from build123d import *

# Parameters (mm, degrees)
BOSS_EXTRUDE1_DEPTH = 4
SKETCH2_R           = 1
CUT_EXTRUDE1_DEPTH  = 5


with BuildPart() as part:
    # Sketch1 → Boss-Extrude1 (new body)
    with BuildSketch(Plane(origin=(0, 0, 0), x_dir=(1, 0, 0), z_dir=(0, 1, 0))):
        with BuildLine():
            Line((-32, -13), (32, -13))
            ThreePointArc((32, -13), (34.121320344, -12.121320344), (35, -10))
            Line((35, -10), (35, 10))
            ThreePointArc((35, 10), (34.121320344, 12.121320344), (32, 13))
            Line((32, 13), (-32, 13))
            ThreePointArc((-32, 13), (-34.121320344, 12.121320344), (-35, 10))
            Line((-35, 10), (-35, -10))
            ThreePointArc((-35, -10), (-34.121320344, -12.121320344), (-32, -13))
        make_face()
        with BuildLine():
            Line((-26.749817226, -6), (26.749817226, -6))
            ThreePointArc((26.749817226, -6), (28.871137569, -5.121320344), (29.749817226, -3))
            Line((29.749817226, -3), (29.749817226, 3))
            ThreePointArc((29.749817226, 3), (28.871137569, 5.121320344), (26.749817226, 6))
            Line((26.749817226, 6), (-26.749817226, 6))
            ThreePointArc((-26.749817226, 6), (-28.871137569, 5.121320344), (-29.749817226, 3))
            Line((-29.749817226, 3), (-29.749817226, -3))
            ThreePointArc((-29.749817226, -3), (-28.871137569, -5.121320344), (-26.749817226, -6))
        make_face(mode=Mode.SUBTRACT)
        with BuildLine():
            Line((-28.749817226, 11.5), (28.749817226, 11.5))
            ThreePointArc((28.749817226, 11.5), (29.456924007, 11.207106781), (29.749817226, 10.5))
            Line((29.749817226, 10.5), (29.749817226, 9.5))
            ThreePointArc((29.749817226, 9.5), (29.456924007, 8.792893219), (28.749817226, 8.5))
            Line((28.749817226, 8.5), (-28.749817226, 8.5))
            ThreePointArc((-28.749817226, 8.5), (-29.456924007, 8.792893219), (-29.749817226, 9.5))
            Line((-29.749817226, 9.5), (-29.749817226, 10.5))
            ThreePointArc((-29.749817226, 10.5), (-29.456924007, 11.207106781), (-28.749817226, 11.5))
        make_face(mode=Mode.SUBTRACT)
        with BuildLine():
            Line((-29.749817226, -10.5), (-29.749817226, -9.5))
            ThreePointArc((-29.749817226, -9.5), (-29.456924007, -8.792893219), (-28.749817226, -8.5))
            Line((-28.749817226, -8.5), (28.749817226, -8.5))
            ThreePointArc((28.749817226, -8.5), (29.456924007, -8.792893219), (29.749817226, -9.5))
            Line((29.749817226, -9.5), (29.749817226, -10.5))
            ThreePointArc((29.749817226, -10.5), (29.456924007, -11.207106781), (28.749817226, -11.5))
            Line((28.749817226, -11.5), (-28.749817226, -11.5))
            ThreePointArc((-28.749817226, -11.5), (-29.456924007, -11.207106781), (-29.749817226, -10.5))
        make_face(mode=Mode.SUBTRACT)
    extrude(amount=BOSS_EXTRUDE1_DEPTH)

    # Sketch2 → Cut-Extrude1 (cut)
    with BuildSketch(Plane(origin=(35, 0, 0), x_dir=(0, 0, -1), z_dir=(1, 0, 0))):
        with Locations((-8, 2)):
            Circle(SKETCH2_R)
        with Locations((8, 2)):
            Circle(SKETCH2_R)
    extrude(amount=-CUT_EXTRUDE1_DEPTH, mode=Mode.SUBTRACT)


solid = part.part
The model under review builds one solid part; all positions refer to its coordinate system, in mm. A direction names the side the tool comes from. Give positions to 0.01 mm unless a question says otherwise; leave off trailing zeros. Write each loop counter-clockwise with the first axis right and the second up, starting at its lowest first coordinate (ties: lowest second). Pieces come first, ordered by that corner, then holes. Notation, with made-up numbers: M 88.5,84.5 L 143.5,84.5 A30 ccw 143.5,107.5 Z; hole C 30,-28.75 d11. An arc over 180 degrees is marked long. One line per question, with ' | ' between items. Start each with the question number.
Item 1: Wall thickness on line 1 (Z direction, x = 13, y = 2.1); line 2 (Y direction, x = 32.4, z = 8); line 3 (X direction, y = 3.1, z = -3.25): over which ranges is each line inside the solid? List them lowest first. Write a range as from..to.
Item 2: We need section D-D on y = 2. Give the number of separate pieces and of enclosed holes in the cut face, plus the area to 3 significant figures.
Item 3: For pin 1 (1.6 mm diameter, centred on y = 2, z = -8, fed in from +X), flat-tipped, find the tip position at first contact; note if it passes through.
Item 4: For faces 1 (the cylindrical face through (-34.14, 1.97, 12.1)), 2 (the flat face through (0, 2, -8.5)), list the 3-axis set-ups (+Z, -Z, +X, -X, +Y, -Y) from which the entire face can be reached by the end or side of a thin tool; tool diameter is ignored.
Item 5: We need section A-A on x = 19. Write out the cut boundary in (y, z).
Item 6: Draft analysis for pull direction Y (two halves, no side actions). For faces 3 (the flat face through (30, 2, -8)), 4 (the flat face through (0, 4, 8)), 5 (the flat face through (30, 2, 8)), 6 (the flat face through (35, 2, 0)), state which applies: released by +Y, released by -Y, zero draft, split by the parting line, or undercut.
Item 7: We need section B-B on z = -2. Write out the cut boundary in (x, y).
Item 8: We need section C-C on x = -28. Write out the cut boundary in (y, z).
Results found:
1) line 1: z = -13..-11.5, -8.5..-6, 6..8.5, 11.5..13 | line 2: y = 0..1, 3..4 | line 3: x = -35..-29.74, 29.74..35
2) separate pieces: 1 | enclosed holes: 3 | area: 731 mm2
3) pin 1: stops at x = 30
4) face 1: +Z, -X, +Y, -Y | face 2: +Y, -Y
5) outline: M 0,-13 L 4,-13 L 4,-11.5 L 0,-11.5 Z; M 0,-8.5 L 4,-8.5 L 4,-6 L 0,-6 Z; M 0,6 L 4,6 L 4,8.5 L 0,8.5 Z; M 0,11.5 L 4,11.5 L 4,13 L 0,13 Z
6) face 3: undercut | face 4: released by +Y | face 5: undercut | face 6: zero draft
7) outline: M -35,0 L -29.75,0 L -29.75,4 L -35,4 Z; M 29.75,0 L 35,0 L 35,4 L 29.75,4 Z
8) outline: M 0,-13 L 4,-13 L 4,-11.5 L 0,-11.5 Z; M 0,-8.5 L 4,-8.5 L 4,-5.73 L 0,-5.73 Z; M 0,5.73 L 4,5.73 L 4,8.5 L 0,8.5 Z; M 0,11.5 L 4,11.5 L 4,13 L 0,13 Z
